Read the model definition and answer for the solid it produces. Units are mm, in the model's axes. Face numbers are marked on the shaded views. A direction names the side the tool comes from. Give positions to 0.01 mm unless a question says otherwise; leave off trailing zeros. Order: outer loops, then holes, each group sorted by start corner. A loop starts at its lowest first (then second) coordinate and runs counter-clockwise, first axis right, second up. Notation, with made-up numbers: M -15,21 L 3,21 A20 ccw 3,27 Z; hole C -35,58.5 d3. An arc over 180 degrees is marked long. Write item = value, one per line. Start each with the question number.
from build123d import *

# Parameters (mm, degrees)
F1_DEPTH = 25.4
F2_W     = 15.24
F2_H     = 14.986
F2_W_2   = 48.74875
F3_DEPTH = 76.2
F5_DEPTH = 25.4


with BuildPart() as f1:
    # F0 (on Top) → F1 (new body)
    with BuildSketch(Plane.XY):
        with BuildLine():
            Line((1.640223, 29.21), (-30.871777, 29.21))
            Line((-30.871777, 29.21), (-30.871777, 19.05))
            Line((-30.871777, 19.05), (-37.475777, 19.05))
            Line((-37.475777, 19.05), (-37.475777, -19.05))
            Line((-37.475777, -19.05), (-30.871777, -19.05))
            Line((-30.871777, -19.05), (-30.871777, -29.21))
            Line((-30.871777, -29.21), (1.640223, -29.21))
            Line((1.640223, -29.21), (49.900223, -21.59))
            Line((49.900223, -21.59), (49.900223, -9.906))
            Line((49.900223, -9.906), (21.452223, -9.906))
            ThreePointArc((21.452223, -9.906), (11.546223, 0), (21.452223, 9.906))
            Line((21.452223, 9.906), (49.900223, 9.906))
            Line((49.900223, 9.906), (49.900223, 21.59))
            Line((49.900223, 21.59), (1.640223, 29.21))
        make_face()
    extrude(amount=F1_DEPTH)

    # F2 (on face) → F3 (cut)
    with BuildSketch(Plane.XZ.offset(29.21)):
        with Locations((-5.979777, 17.907)):
            Rectangle(F2_W, F2_H)
        with Locations((26.014598, 17.907)):
            Rectangle(F2_W_2, F2_H)
    extrude(amount=-F3_DEPTH, mode=Mode.SUBTRACT)

    # F4 (on face) → F5 (cut)
    with BuildSketch(Plane.YZ.offset(-13.599777)):
        Polygon((-29.21, 14.224), (-9.8526, 25.4), (-29.21, 25.4), align=None)
        Polygon((29.21, 25.4), (9.8526, 25.4), (29.21, 14.224), align=None)
    extrude(amount=-F5_DEPTH, mode=Mode.SUBTRACT)


solid = f1.part
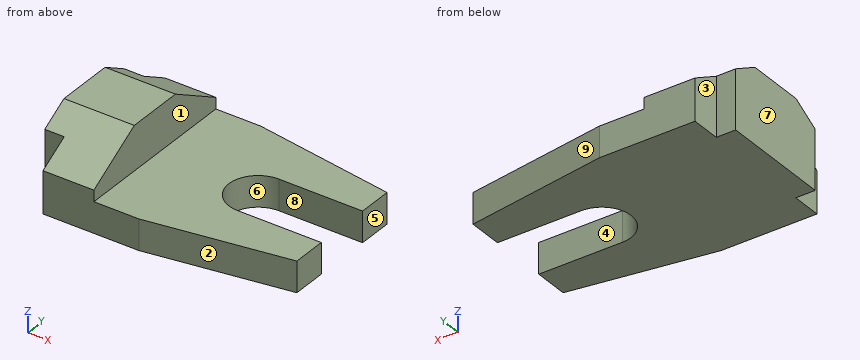
1) For the marked faces 1, 2, 3, 4 and 5, determine the directions among +Z, -Z, +X, -X, +Y, -Y from which every point of the face is accessible in a straight line to the end or side of a thin tool.
2) For a pull along Y with two mould halves and no side action, classify the marked faces 6, 7, 8 and 9 as pulls with the +Y half, pulls with the -Y half, needs draft (parallel to the pull), parting line crosses it, or undercut.
3) Find section D-D on y = 0. Determine the outline of the cut face in (x, z), plus the area to 3 significant figures.
4) Find section A-A on x = 25. Determine the outline of the cut face in (y, z).
5) Each of these flat-tipped pins is pushed along its axis until it touches: P1, Ø5, axis at x = 34, z = 5, coming from the +Y side; P2, Ø1.5, axis at x = -4, y = 23.5, coming from the +Z side; P3, Ø8, axis at x = 12.5, z = 10.5, coming from the -Y side. Where does it stop, or does it pass through?
6) Find section B-B on z = 11.5. Determine the outline of the cut face in (x, y).
7) Find the intervals of material crossed by probe 1 along X at (y, z) = (-1, 23.25); probe 2 along Z at (x, y) = (18, -20.5); probe 3 along Y at (x, z) = (13, 10), in increasing order. Write a range as [from, to].
8) Find section C-C on x = -15. Determine the outline of the cut face in (y, z), plus the area to 3 significant figures.
Numbers:
q1.face_1 = +Z, +X, +Y, -Y
q1.face_2 = +Z, -Z, +X, -Y
q1.face_3 = +Z, -Z, -X, +Y
q1.face_4 = +Z, -Z, +X
q1.face_5 = +Z, -Z, +X, +Y, -Y
q2.face_6 = undercut
q2.face_7 = needs draft
q2.face_8 = undercut
q2.face_9 = pulls with the +Y half
q3.outline = M -37.48,0 L 11.55,0 L 11.55,10.41 L -13.6,10.41 L -13.6,25.4 L -37.48,25.4 Z
q3.area = 868 mm2
q4.outline = M -25.52,0 L -9.91,0 L -9.91,10.41 L -25.52,10.41 Z; M 9.91,0 L 25.52,0 L 25.52,10.41 L 9.91,10.41 Z
q5.P1 = 24.5
q5.P2 = 10.41
q5.P3 = -28.13
q6.outline = M -37.48,-19.05 L -30.87,-19.05 L -30.87,-29.21 L -13.6,-29.21 L -13.6,29.21 L -30.87,29.21 L -30.87,19.05 L -37.48,19.05 Z
q7.probe_1 = [-37.48, -13.6]
q7.probe_2 = [0, 10.41]
q7.probe_3 = [-27.42, -5.17], [5.17, 27.42]
q8.outline = M -29.21,0 L 29.21,0 L 29.21,14.22 L 9.85,25.4 L -9.85,25.4 L -29.21,14.22 Z
q8.area = 1,270 mm2
